Input: part model. Units: mm. Frame: model coordinates. A direction names the side the tool comes from. Give positions to 0.01 mm unless a question says otherwise; leave off trailing zeros. Order: outer loops, then holes, each group sorted by start corner. A loop starts at its lowest first (then second) coordinate and runs counter-clockwise, first axis right, second up. Notation, with made-up numbers: (-27.5, 20.25) - (17.5, 20.25) arc R5 cw to (17.5, 26.25) - close; hole circle Ø1 at (55, -31.5). An arc over 180 degrees is marked (long way). Use a Markdown table: item, result.
from build123d import *

# Parameters (mm, degrees)
F1_DEPTH = 2
F2_SIZE  = 1
F3_R     = 0.4


with BuildPart() as f1:
    # F0 (on Top) → F1 (new body)
    with BuildSketch(Plane.XY):
        with BuildLine():
            Line((-1.338212, 64), (-1.338212, 5.848862))
            ThreePointArc((-1.338212, 5.848862), (0, -6), (1.338212, 5.848862))
            Line((1.338212, 5.848862), (1.338212, 64))
            ThreePointArc((1.338212, 64), (1.898957, 65.837607), (3.390126, 67.049072))
            Line((3.390126, 67.049072), (0, 80))
            Line((0, 80), (-3.390126, 67.049072))
            ThreePointArc((-3.390126, 67.049072), (-1.898957, 65.837607), (-1.338212, 64))
        make_face()
        with BuildLine():
            ThreePointArc((2.999796, 0.034951), (2.999949, 0.017476), (3, 0))
            ThreePointArc((3, 0), (-2.999949, -0.017476), (2.999796, 0.034951))
        make_face(mode=Mode.SUBTRACT)
    extrude(amount=F1_DEPTH)

    # F2
    f2_edges = [f1.edges().sort_by_distance(p)[0] for p in [
        (0, -6, 2),
    ]]
    chamfer(f2_edges, length=F2_SIZE)

    # F3
    f3_edges = [f1.edges().sort_by_distance(p)[0] for p in [
        (1.338212, 34.924431, 2),
        (-1.338212, 34.924431, 2),
        (1.695063, 73.524536, 2),
        (-1.695063, 73.524536, 2),
        (1.898957, 65.837607, 2),
        (-1.898957, 65.837607, 2),
    ]]
    fillet(f3_edges, radius=F3_R)


solid = f1.part
1. Pin query (flat end, axial travel): pin 1 (0.8 mm diameter, centred on y = 41.5, z = 0.5, fed in from -X); pin 2 (0.8 mm diameter, centred on y = 31, z = 0.5, fed in from +X). Return the tip coordinate at first contact, or that it passes through.
Response:
| item | result |
|---|---|
| pin 1 | stops at x = -1.34 |
| pin 2 | stops at x = 1.34 |
2. Material intervals for line 1 along X through (y, z) = (38.5, 1); line 2 along X through (y, z) = (2, 1); line 3 along X through (y, z) = (66, 1.9), sorted ascending.
Response:
| item | result |
|---|---|
| line 1 | x = -1.34 to 1.34 |
| line 2 | x = -5.66 to -2.24, 2.24 to 5.66 |
| line 3 | x = -1.85 to 1.85 |
3. Section query A-A (y = 49.5). Return loops of the section in (x, z).
Response:
| item | result |
|---|---|
| outline | (-1.34, 0) - (1.34, 0) - (1.34, 1.6) arc R0.4 ccw to (0.94, 2) - (-0.94, 2) arc R0.4 ccw to (-1.34, 1.6) - close |
4. Mould query, pull axis Y, two halves, no side actions, for faces 1 (the face through (1.72, 73.43, 0.79)), 2 (the face through (-0.213, -5.155, 1.84)), 3 (the face through (-1.914, 65.86, 0.789)), 4 (the face through (0, 31, 0)). Classes: pulls with the +Y half, pulls with the -Y half, needs draft (parallel to the pull), parting line crosses it, or undercut.
Response:
| item | result |
|---|---|
| face 1 | pulls with the +Y half |
| face 2 | undercut |
| face 3 | undercut |
| face 4 | needs draft |
5. Set-up query: faces 5 (the face through (1.88, 65.81, 0.79)), 6 (the face through (-1.338, 35, 1)), 7 (the face through (-3, 0, 1)). Return all of +Z, -Z, +X, -X, +Y, -Y with unobstructed straight access to the full face (end or side cutting, diameter ignored); none if empty.
Response:
| item | result |
|---|---|
| face 5 | +Z, -Z, +X |
| face 6 | +Z, -Z, -X |
| face 7 | +Z, -Z |
